from build123d import *

# Parameters (mm, degrees)
F0_R     = 4
F0_R_2   = 3.4982450121
F0_R_3   = 3.0047107059
F1_DEPTH = 1
F2_R     = 2.9066223448
F2_R_2   = 2.45
F3_DEPTH = 2
F4_R     = 2.5488613676
F5_DEPTH = 1.5
F7_D     = 3
F7_DEPTH = 2
F7_TIP   = 0.9012909285


with BuildPart() as f1:
    # F0 (on Front) → F1 (new body)
    with BuildSketch(Plane.XZ):
        with Locations((-18.8527759165, 9.8558971658)):
            Circle(F0_R)
        with Locations((-18.8527759165, 9.8558971658)):
            Circle(F0_R_2, mode=Mode.SUBTRACT)
        with Locations((-18.8527759165, 9.8558971658)):
            Circle(F0_R_2)
        with Locations((-18.8527759165, 9.8558971658)):
            Circle(F0_R_3, mode=Mode.SUBTRACT)
        with Locations((-18.8527759165, 9.8558971658)):
            Circle(F0_R_3)
    extrude(amount=F1_DEPTH)

    # F2 (on face) → F3 (join)
    with BuildSketch(Plane.XZ.offset(1)):
        with Locations((-18.8527759165, 9.8558971658)):
            Circle(F2_R)
        with Locations((-18.8527759165, 9.8558971658)):
            Circle(F2_R_2, mode=Mode.SUBTRACT)
    extrude(amount=F3_DEPTH)

    # F4 (on face) → F5 (join)
    with BuildSketch(Plane(origin=(0, 0, 0), x_dir=(-1, 0, 0), z_dir=(0, 1, 0))):
        with Locations((18.8527759165, 9.8558971658)):
            Circle(F4_R)
    extrude(amount=F5_DEPTH)

    # F7 (one way)
    with BuildSketch(Plane(origin=(0, 0, 0), x_dir=(1, 0, 0), z_dir=(0, 1, 0))):
        with Locations((-18.891595304, -9.8473792896)):
            Circle(F7_D / 2)
    extrude(amount=-F7_DEPTH, mode=Mode.SUBTRACT)
    with Locations(Plane(origin=(0, 0, 0), x_dir=(1, 0, 0), z_dir=(0, 1, 0))):
        with Locations((-18.891595304, -9.8473792896)):
            with Locations((0, 0, -(F7_DEPTH + F7_TIP / 2))):  # 118° drill point
                Cone(0, F7_D / 2, F7_TIP, mode=Mode.SUBTRACT)


solid = f1.part
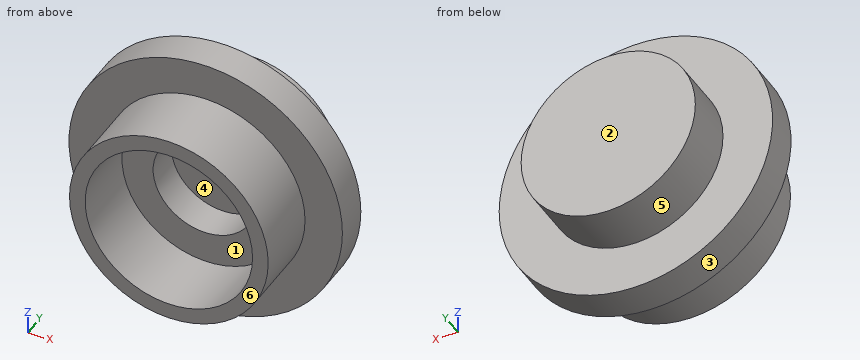
Could you check a few things on this model? Use its own coordinates, in mm. Face numbers are marked on the shaded views. A direction names the side the tool comes from. Give positions to 0.01 mm unless a question says otherwise; leave off trailing zeros. Loops run counter-clockwise (first coordinate to the right, second up) from the corner with the lowest first, then second, coordinate; pieces in that order, holes last. Notation, with made-up numbers: (-28, -18) -> (28, -18) arc R24 cw to (28, 10) -> close; hole circle Ø6 at (60, 67). An arc over 180 degrees is marked (long way). Return JSON: item names as keys, results as strings.
Item 1: I need wall thicknesses on L1, parallel to Y at x = -17, z = 12.25; L2, parallel to X at y = -1.15, z = 9; L3, parallel to Y at x = -18, z = 8. Which ranges of each line are inside material? Lowest first, please. Write a range as from..to.
Geometry results:
{"L1": "y = -1..0", "L2": "x = -21.63..-21.15, -16.56..-16.08", "L3": "y = -1..1.5"}
Item 2: If we section it at A-A on x = -17.25: List the corners of the cut face in (y, z) for me.
Geometry results:
{"outline": "(-3, 7.43) -> (-1, 7.43) -> (-1, 6.19) -> (0, 6.19) -> (0, 7.87) -> (1.5, 7.87) -> (1.5, 11.84) -> (0, 11.84) -> (0, 13.52) -> (-1, 13.52) -> (-1, 12.28) -> (-3, 12.28) -> (-3, 11.71) -> (-1, 11.71) -> (-1, 8) -> (-3, 8) -> close"}
Item 3: We'd pull the mould along X, two halves only. Please class the marked faces 1, 2 and 3: +X half, -X half, draft (parallel to the pull), parting line (faces both ways), or undercut.
Geometry results:
{"face 1": "undercut", "face 2": "draft", "face 3": "parting line"}
Item 4: If we section it at B-B on z = 9: List the corners of the cut face in (x, y) for me, plus the area to 3 significant figures.
Geometry results:
{"outline": "(-22.76, -1) -> (-21.63, -1) -> (-21.63, -3) -> (-21.15, -3) -> (-21.15, -1) -> (-20.13, -1) -> (-20.13, 0) -> (-17.65, 0) -> (-17.65, -1) -> (-16.56, -1) -> (-16.56, -3) -> (-16.08, -3) -> (-16.08, -1) -> (-14.95, -1) -> (-14.95, 0) -> (-16.45, 0) -> (-16.45, 1.5) -> (-21.25, 1.5) -> (-21.25, 0) -> (-22.76, 0) -> close", "area": "14.5 mm²"}
Item 5: I'm going to push a flat-ended pin straight in: pin 1 (3.5 mm diameter, centred on x = -18.89, z = 9.85, fed in from -Y). Where does the tip first touch, or does it pass through?
Geometry results:
{"pin 1": "stops at y = -1"}
Item 6: If we section it at C-C on x = -20.5: List the corners of the cut face in (y, z) for me, plus the area to 3 significant figures.
Geometry results:
{"outline": "(-3, 7.46) -> (-1, 7.46) -> (-1, 6.21) -> (0, 6.21) -> (0, 7.91) -> (1.5, 7.91) -> (1.5, 11.8) -> (0, 11.8) -> (0, 13.5) -> (-1, 13.5) -> (-1, 12.25) -> (-3, 12.25) -> (-3, 11.67) -> (-1, 11.67) -> (-1, 8.04) -> (-3, 8.04) -> close", "area": "15.5 mm²"}
Item 7: Which directions (+Z, -Z, +X, -X, +Y, -Y) give clear straight access to the entire face, cutting with the end or side of a thin tool? Please do the marked faces 4, 5 and 6.
Geometry results:
{"face 4": "-Y", "face 5": "+Y", "face 6": "+Z, -Z, +X, -X, -Y"}
Item 8: If we section it at D-D on y = -1.45: List the corners of the cut face in (x, z) for me, plus the area to 3 significant figures.
Geometry results:
{"outline": "circle Ø5.81 at (-18.85, 9.86); hole circle Ø4.9 at (-18.85, 9.86)", "area": "7.68 mm²"}
